Print and shaded views of the part. All mm, measured from the part's lowest x, y and z. A direction names the side the tool comes from. Round coordinates to 2 decimals unless told otherwise and drop trailing zeros. Order: outer loops, then holes, each group sorted by start corner. A loop starts at its lowest first (then second) coordinate and runs counter-clockwise, first axis right, second up. Notation, with made-up numbers: (-6, 11.25) - (21, 11.25) arc R28 cw to (21, 43.25) - close; hole circle Ø6 at (-15, -24.75). An arc over 180 degrees is marked (long way). Write item = value, one per line.
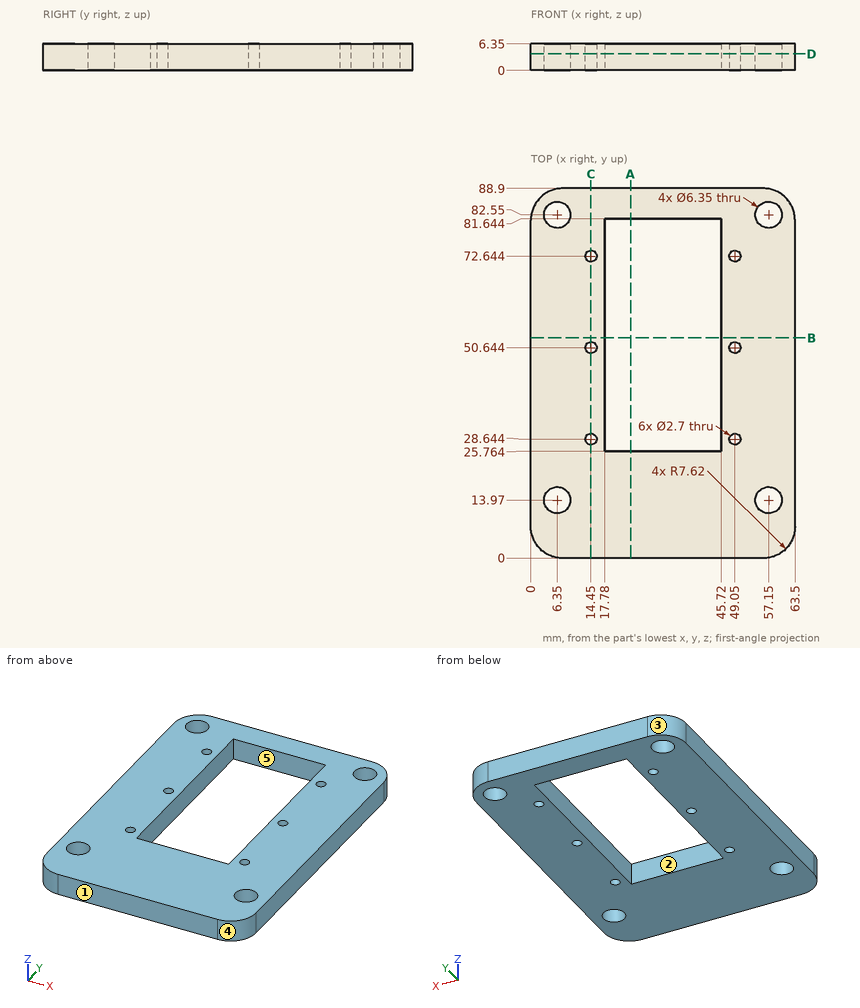
(1) Drop a flat-ended pin along its axis: pin 1 (1.6 mm diameter, centred on x = 14.45, y = 28.644, fed in from -Z). Give the stop position or say it passes through.
Solved:
pin_1 = through
(2) Tool access for the marked faces 1 and 2: list every direction of +Z, -Z, +X, -X, +Y, -Y with a clear straight run to the whole face (end or side of a thin tool).
Solved:
face_1 = +Z, -Z, +X, -X, -Y
face_2 = +Z, -Z
(3) Band-saw the part on A-A on x = 24. List the corners of the cut face in (y, z).
Solved:
outline = (0, 0) - (25.76, 0) - (25.76, 6.35) - (0, 6.35) - close; (81.64, 0) - (88.9, 0) - (88.9, 6.35) - (81.64, 6.35) - close
(4) Pull direction X, two halves, no side cores. Call the marked faces 3, 4 and 5: released by +X, released by -X, zero draft, split by the parting line, or undercut.
Solved:
face_3 = released by -X
face_4 = released by +X
face_5 = undercut
(5) Band-saw the part on C-C on x = 14.45. List the corners of the cut face in (y, z).
Solved:
outline = (0, 0) - (27.29, 0) - (27.29, 6.35) - (0, 6.35) - close; (29.99, 0) - (49.29, 0) - (49.29, 6.35) - (29.99, 6.35) - close; (51.99, 0) - (71.29, 0) - (71.29, 6.35) - (51.99, 6.35) - close; (73.99, 0) - (88.9, 0) - (88.9, 6.35) - (73.99, 6.35) - close
(6) Probe line 1 along Y through (x, z) = (14.45, 4.25); line 2 along Y through (x, z) = (29.5, 5.5); line 3 along X through (y, z) = (77, 0.75). List the from-to ranges inside material, lowest first.
Solved:
line_1 = 0 to 27.29, 29.99 to 49.29, 51.99 to 71.29, 73.99 to 88.9
line_2 = 0 to 25.76, 81.64 to 88.9
line_3 = 0 to 17.78, 45.72 to 63.5
(7) Band-saw the part on B-B on y = 53. List the corners of the cut face in (x, z).
Solved:
outline = (0, 0) - (17.78, 0) - (17.78, 6.35) - (0, 6.35) - close; (45.72, 0) - (63.5, 0) - (63.5, 6.35) - (45.72, 6.35) - close
(8) Band-saw the part on D-D on z = 4. Count the separate pieces of the cut face and the enclosed holes in it, plus the area to 3 significant figures.
Solved:
separate_pieces = 1
enclosed_holes = 11
area = 3,870 mm²
